Here's how the part is built. I have some questions about the finished solid (model axes, mm). Face numbers are marked on the shaded views. Round coordinates to 2 decimals unless told otherwise and drop trailing zeros. Write each loop counter-clockwise with the first axis right and the second up, starting at its lowest first coordinate (ties: lowest second). Pieces come first, ordered by that corner, then holes. Notation, with made-up numbers: (28, 41.25) - (77, 41.25) arc R29 cw to (77, 61.25) - close; hole circle Ø1 at (1.5, -6). An arc over 180 degrees is marked (long way). One line per question, with ' | ' between items. Start each with the question number.
(1) Will these pins go through, and if not, where does the flat tip stop? pin 1 (8 mm diameter, centred on x = 20.5, z = 24, fed in from -Y); pin 2 (1 mm diameter, centred on x = 13.5, y = -3, fed in from -Z) (3 decimals); pin 3 (1.6 mm diameter, centred on x = 33.5, z = 33.5, fed in from -Y).
(2) If I drill on L1, parallel to Z at x = -7, y = -1.75; L2, parallel to X at y = -7, z = -43.5; L3, parallel to Z at x = 8.5, y = -0.5, over which ranges is the centre line in solid material (lowest first)?
(3) Imagine slicing it at D-D (x = 4). Write out the boundary of the cut face in (y, z), plus the area to 3 significant figures.
(4) Imagine slicing it at A-A (y = -5.5). Write out the boundary of the cut face in (x, z).
(5) Thinking about a two-plate mould opening in X: for the marked faces 1 and 2, which applies, pulls with the +X half, pulls with the -X half, needs draft (parallel to the pull), parting line crosses it, or undercut?
(6) Imagine slicing it at C-C (z = -20). Write out the boundary of the cut face in (x, y), plus the area to 3 significant figures.
(7) Imagine slicing it at B-B (x = -3.5). Write out the boundary of the cut face in (y, z), plus the area to 3 significant figures.
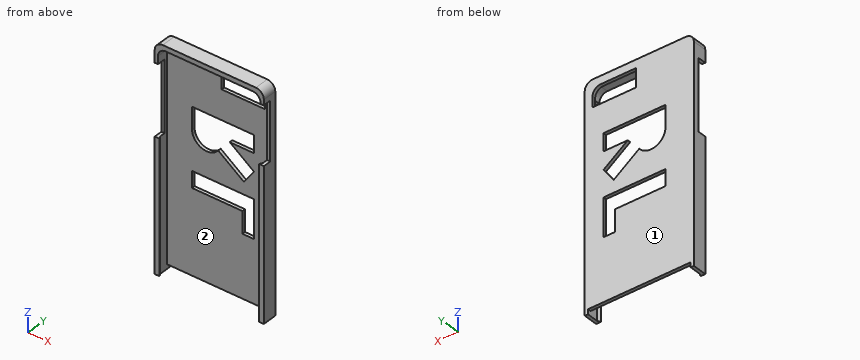
from build123d import *

# Parameters (mm, degrees)
F1_DEPTH  = 2
F2_DEPTH  = 9
F3_W      = 5.0319702644
F3_H      = 36.4959277213
F4_DEPTH  = 5
F5_W      = 5.2322996128
F5_H      = 44.2271307111
F6_DEPTH  = 5
F8_DEPTH  = 10
F9_R      = 5.0696184715
F10_DEPTH = 25
F11_W     = 1.8213601708
F11_H     = 94.6240146787
F12_DEPTH = 1
F13_W     = 1.82136
F13_H     = 82.468239698
F14_DEPTH = 1
F16_DEPTH = 95
F18_DEPTH = 85


with BuildPart() as f1:
    # F0 (on Front) → F1 (new body)
    with BuildSketch(Plane.XZ):
        with BuildLine():
            Line((-32.15, -67.5050175221), (32.15, -67.5050175221))
            Line((32.15, -67.5050175221), (32.15, 60.9949824779))
            ThreePointArc((32.15, 60.9949824779), (30.6855339059, 64.5305163838), (27.15, 65.9949824779))
            Line((27.15, 65.9949824779), (-27.15, 65.9949824779))
            ThreePointArc((-27.15, 65.9949824779), (-30.6855339059, 64.5305163838), (-32.15, 60.9949824779))
            Line((-32.15, 60.9949824779), (-32.15, -67.5050175221))
        make_face()
    extrude(amount=F1_DEPTH)

    # F0 (on Front) → F2 (join)
    with BuildSketch(Plane.XZ):
        with BuildLine():
            Line((32.15, -70.5050175221), (34.15, -70.5050175221))
            Line((34.15, -70.5050175221), (34.15, 63.9949824779))
            ThreePointArc((34.15, 63.9949824779), (32.6855339059, 67.5305163838), (29.15, 68.9949824779))
            Line((29.15, 68.9949824779), (-29.15, 68.9949824779))
            ThreePointArc((-29.15, 68.9949824779), (-32.6855339059, 67.5305163838), (-34.15, 63.9949824779))
            Line((-34.15, 63.9949824779), (-34.15, -70.5050175221))
            Line((-34.15, -70.5050175221), (-32.15, -70.5050175221))
            Line((-32.15, -70.5050175221), (-32.15, -67.5050175221))
            Line((-32.15, -67.5050175221), (-32.15, 60.9949824779))
            ThreePointArc((-32.15, 60.9949824779), (-30.6855339059, 64.5305163838), (-27.15, 65.9949824779))
            Line((-27.15, 65.9949824779), (27.15, 65.9949824779))
            ThreePointArc((27.15, 65.9949824779), (30.6855339059, 64.5305163838), (32.15, 60.9949824779))
            Line((32.15, 60.9949824779), (32.15, -67.5050175221))
            Line((32.15, -67.5050175221), (32.15, -70.5050175221))
        make_face()
    extrude(amount=F2_DEPTH)

    # F3 (on face) → F4 (cut)
    with BuildSketch(Plane.YZ.offset(34.15)):
        with Locations((-6.4840148678, 42.3669610173)):
            Rectangle(F3_W, F3_H)
    extrude(amount=-F4_DEPTH, mode=Mode.SUBTRACT)

    # F5 (on face) → F6 (cut)
    with BuildSketch(Plane(origin=(-34.15, 0, 0), x_dir=(0, -1, 0), z_dir=(-1, 0, 0))):
        with Locations((6.3838501936, 34.0767875314)):
            Rectangle(F5_W, F5_H)
    extrude(amount=-F6_DEPTH, mode=Mode.SUBTRACT)

    # F7 (on face) → F8 (cut)
    with BuildSketch(Plane.XZ.offset(2)):
        with BuildLine():
            Line((2.180054551, 63.9047697186), (2.180054551, 52.2672943771))
            Line((2.180054551, 52.2672943771), (29.2200669646, 52.2672943771))
            Line((29.2200669646, 52.2672943771), (29.2200669646, 58.9047697186))
            ThreePointArc((29.2200669646, 58.9047697186), (27.7556008706, 62.4403036246), (24.2200669646, 63.9047697186))
            Line((24.2200669646, 63.9047697186), (2.180054551, 63.9047697186))
        make_face()
    extrude(amount=-F8_DEPTH, mode=Mode.SUBTRACT)

    # F9 (on face) → F10 (cut)
    with BuildSketch(Plane.XZ.offset(2)):
        Polygon((22.451505065, -4.7073736787), (-16.3505785167, -4.7073736787), (-16.3505785167, -14.9441054091), (15.2370482683, -14.9441054091), (15.2370482683, -28.5930782557), (22.451505065, -28.5930782557), align=None)
        with BuildLine():
            Line((22.451505065, 33.8022336364), (-16.3505785167, 33.8022336364))
            Line((-16.3505785167, 33.8022336364), (-16.3505785167, 20.1532579958))
            ThreePointArc((-16.3505785167, 20.1532579958), (-10.1403629568, 11.5351459717), (0, 14.6992684827))
            Line((0, 14.6992684827), (16.0316545011, 2.9838289004))
            Line((16.0316545011, 2.9838289004), (22.451505065, 11.7688877508))
            Line((22.451505065, 11.7688877508), (7.2426483966, 22.8830520064))
            Line((7.2426483966, 22.8830520064), (22.451505065, 22.8830520064))
            Line((22.451505065, 22.8830520064), (22.451505065, 33.8022336364))
        make_face()
        with Locations((-7.3812524788, 24.0529645234)):
            Circle(F9_R, mode=Mode.SUBTRACT)
        with Locations((-7.3812524788, 24.0529645234)):
            Circle(F9_R)
    extrude(amount=-F10_DEPTH, mode=Mode.SUBTRACT)

    # F11 (on face) → F12 (join)
    with BuildSketch(Plane(origin=(32.15, 0, 0), x_dir=(0, -1, 0), z_dir=(-1, 0, 0))):
        with Locations((8.0893199146, -23.1930101828)):
            Rectangle(F11_W, F11_H)
    extrude(amount=F12_DEPTH)

    # F13 (on face) → F14 (join)
    with BuildSketch(Plane.YZ.offset(-32.15)):
        with Locations((-8.08932, -29.2708976731)):
            Rectangle(F13_W, F13_H)
    extrude(amount=F14_DEPTH)

    # F15 (on face) → F16 (cut)
    with BuildSketch(Plane(origin=(0, 0, -70.5050175221), x_dir=(1, 0, 0), z_dir=(0, 0, -1))):
        Polygon((31.15, 7.1786398292), (32.15, 7.1786398292), (31.15, 9), align=None)
    extrude(amount=-F16_DEPTH, mode=Mode.SUBTRACT)

    # F17 (on face) → F18 (cut)
    with BuildSketch(Plane(origin=(0, 0, -70.5050175221), x_dir=(1, 0, 0), z_dir=(0, 0, -1))):
        Polygon((-31.15, 9), (-32.15, 7.17864), (-31.15, 7.17864), align=None)
    extrude(amount=-F18_DEPTH, mode=Mode.SUBTRACT)


solid = f1.part
Check sheet entries:
1) pin 1: y = -2 | pin 2: z = 65.995 | pin 3: y = -3.97
2) L1: -67.51 to -14.94, -4.71 to 11.07, 33.8 to 68.99 | L2: -34.15 to -32.15, 32.15 to 34.15 | L3: -67.51 to -14.94, -4.71 to 8.49, 21.96 to 22.88, 33.8 to 52.27, 63.9 to 68.99
3) outline: (-9, 65.99) - (-2, 65.99) - (-2, 63.9) - (0, 63.9) - (0, 68.99) - (-9, 68.99) - close; (-2, -67.51) - (0, -67.51) - (0, -14.94) - (-2, -14.94) - close; (-2, -4.71) - (0, -4.71) - (0, 11.78) - (-2, 11.78) - close; (-2, 33.8) - (0, 33.8) - (0, 52.27) - (-2, 52.27) - close | area: 206 mm^2
4) outline: (-34.15, -70.51) - (-32.15, -70.51) - (-32.15, 11.96) - (-34.15, 11.96) - close; (-34.15, 56.19) - (-32.15, 56.19) - (-32.15, 60.99) arc R5 cw to (-27.15, 65.99) - (27.15, 65.99) arc R5 cw to (32.15, 60.99) - (32.15, 60.61) - (34.15, 60.61) - (34.15, 63.99) arc R5 ccw to (29.15, 68.99) - (-29.15, 68.99) arc R5 ccw to (-34.15, 63.99) - close; (32.15, -70.51) - (34.15, -70.51) - (34.15, 24.12) - (32.15, 24.12) - close
5) face 1: needs draft | face 2: undercut
6) outline: (-34.15, -9) - (-31.15, -9) - (-32.15, -7.18) - (-32.15, -2) - (15.24, -2) - (15.24, 0) - (-34.15, 0) - close; (22.45, -2) - (32.15, -2) - (32.15, -7.18) - (31.15, -9) - (34.15, -9) - (34.15, 0) - (22.45, 0) - close | area: 152 mm^2
7) outline: (-9, 65.99) - (-2, 65.99) - (-2, 33.8) - (0, 33.8) - (0, 68.99) - (-9, 68.99) - close; (-2, -67.51) - (0, -67.51) - (0, -14.94) - (-2, -14.94) - close; (-2, -4.71) - (0, -4.71) - (0, 11.89) - (-2, 11.89) - close | area: 230 mm^2
